Verification items for the finished model (mm, model axes). Face numbers are marked on the shaded views. A direction names the side the tool comes from. Coordinates: 2 decimals unless noted, no trailing zeros. Order: outer loops, then holes, each group sorted by start corner. A loop starts at its lowest first (then second) coordinate and runs counter-clockwise, first axis right, second up. Notation, with made-up numbers: M 79.5,-33.75 L 119.5,-33.75 A11 ccw 119.5,-29.75 Z; hole C 11.25,10 d3. An arc over 180 degrees is marked long. Use one line per item in the form item = value. Start each with the question number.
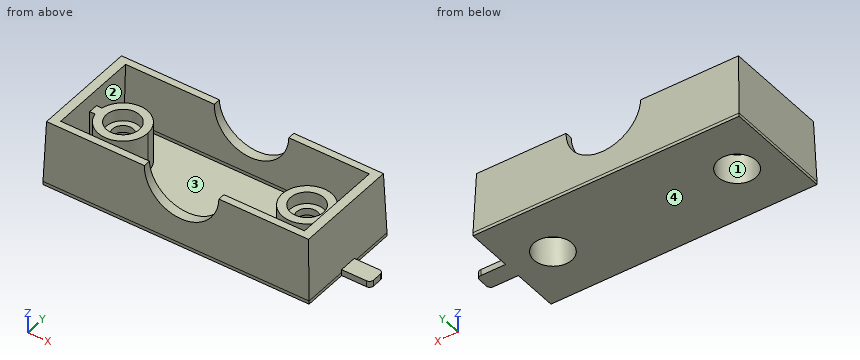
```python
from build123d import *

# Parameters (mm, degrees)
F0_W         = 64.3
F0_H         = 26.3
F1_DEPTH     = 2
F2_W         = 64.3
F2_H         = 26.3
F2_W_2       = 58.9
F2_H_2       = 20.9
F3_DEPTH     = 13.8
F5_DEPTH     = 26.5
F7_DEPTH     = 9.8
F8_R         = 4
F9_DEPTH     = 2.9
F10_R        = 4
F11_DEPTH    = 2.9
F12_R        = 2.5
F13_DEPTH    = 9
F14_R        = 2.5
F15_DEPTH    = 9
F16_R        = 4.6
F17_DEPTH    = 7.2
F18_T1_DEPTH = 102.1483987537
F18_T3_DEPTH = 104.2983987537
F18_T5_DEPTH = 100.1483987537
F19_T1_DEPTH = 53.2490764557
F19_T3_DEPTH = 55.2490764557
F20_W        = 8.1560949282
F20_H        = 4.3
F21_DEPTH    = 1.5
F22_R        = 1


# Not quite as in the source:
# - a fillet or chamfer that OpenCascade refuses, or shapes differently, is made with other operations: its cross-section is extruded or revolved along the edge and cut away or added


with BuildPart() as f1:
    # F0 (on Top) → F1 (new body)
    with BuildSketch(Plane.XY):
        Rectangle(F0_W, F0_H)
    extrude(amount=F1_DEPTH)

    # F2 (on face) → F3 (join)
    with BuildSketch(Plane.XY.offset(2)):
        Rectangle(F2_W, F2_H)
        Rectangle(F2_W_2, F2_H_2, mode=Mode.SUBTRACT)
    extrude(amount=F3_DEPTH)

    # F4 (on face) → F5 (cut)
    with BuildSketch(Plane.XZ.offset(13.15)):
        with BuildLine():
            ThreePointArc((-8, 15.8), (1, 6.8), (10, 15.8))
            Line((10, 15.8), (-8, 15.8))
        make_face()
    extrude(amount=-F5_DEPTH, mode=Mode.SUBTRACT)

    # F6 (on face) → F7 (join)
    with BuildSketch(Plane.XY.offset(2)):
        with BuildLine():
            ThreePointArc((-28.1387604808, -1.15), (-21.6723162131, -5.9721253706), (-16.25, 0))
            ThreePointArc((-16.25, 0), (-21.6723162131, 5.9721253706), (-28.1387604808, 1.15))
            Line((-28.1387604808, 1.15), (-28.1387604808, -1.15))
        make_face()
        with BuildLine():
            Line((-28.1387604808, -1.15), (-28.1387604808, 1.15))
            ThreePointArc((-28.1387604808, 1.15), (-28.25, 0), (-28.1387604808, -1.15))
        make_face()
        with BuildLine():
            ThreePointArc((-28.1387604808, -1.15), (-28.25, 0), (-28.1387604808, 1.15))
            Line((-28.1387604808, 1.15), (-30.8787655085, 1.15))
            Line((-30.8787655085, 1.15), (-30.8787655085, -1.15))
            Line((-30.8787655085, -1.15), (-29.45, -1.15))
            Line((-29.45, -1.15), (-28.1387604808, -1.15))
        make_face()
        with BuildLine():
            ThreePointArc((28.1387604808, -1.15), (28.2221253706, -0.5776837869), (28.25, 0))
            ThreePointArc((28.25, 0), (28.2221253706, 0.5776837869), (28.1387604808, 1.15))
            Line((28.1387604808, 1.15), (28.1387604808, -1.15))
        make_face()
        with BuildLine():
            ThreePointArc((28.1387604808, 1.15), (28.2221253706, 0.5776837869), (28.25, 0))
            ThreePointArc((28.25, 0), (28.2221253706, -0.5776837869), (28.1387604808, -1.15))
            Line((28.1387604808, -1.15), (29.9528725445, -1.15))
            Line((29.9528725445, -1.15), (29.9528725445, 1.15))
            Line((29.9528725445, 1.15), (28.1387604808, 1.15))
        make_face()
        with BuildLine():
            Line((28.1387604808, -1.15), (28.1387604808, 1.15))
            ThreePointArc((28.1387604808, 1.15), (16.25, 0), (28.1387604808, -1.15))
        make_face()
    extrude(amount=F7_DEPTH)

    # F8 (on face) → F9 (cut)
    with BuildSketch(Plane.XY.offset(11.8)):
        with Locations((-22.25, 0)):
            Circle(F8_R)
    extrude(amount=-F9_DEPTH, mode=Mode.SUBTRACT)

    # F10 (on face) → F11 (cut)
    with BuildSketch(Plane.XY.offset(11.8)):
        with Locations((22.25, 0)):
            Circle(F10_R)
    extrude(amount=-F11_DEPTH, mode=Mode.SUBTRACT)

    # F12 (on face) → F13 (cut)
    with BuildSketch(Plane.XY.offset(8.9)):
        with Locations((-22.25, 0)):
            Circle(F12_R)
    extrude(amount=-F13_DEPTH, mode=Mode.SUBTRACT)

    # F14 (on face) → F15 (cut)
    with BuildSketch(Plane.XY.offset(8.9)):
        with Locations((22.25, 0)):
            Circle(F14_R)
    extrude(amount=-F15_DEPTH, mode=Mode.SUBTRACT)

    # F16 (on face) → F17 (cut)
    with BuildSketch(Plane(origin=(0, 0, 0), x_dir=(1, 0, 0), z_dir=(0, 0, -1))):
        with Locations((-22.25, 0)):
            Circle(F16_R)
        with Locations((22.25, 0)):
            Circle(F16_R)
    extrude(amount=-F17_DEPTH, mode=Mode.SUBTRACT)

    # F18: chamfer of 15 x 0.5 on 6 edges, made by hand

    # F18_s2 → F18_t1 (cut)
    with BuildSketch(Plane.YZ.offset(-71.1491993768)):
        Polygon((13.15, 0.8), (12.65, 15.8), (13.15, 15.8), align=None)
        Polygon((-12.65, 15.8), (-13.15, 0.8), (-13.15, 15.8), align=None)
    extrude(amount=F18_T1_DEPTH, mode=Mode.SUBTRACT)

    # F18_s4 → F18_t3 (cut)
    with BuildSketch(Plane.XZ.offset(-52.1491993768)):
        Polygon((32.15, 0.8), (31.65, 15.8), (32.15, 15.8), align=None)
        Polygon((-32.15, 0.8), (-31.65, 15.8), (-32.15, 15.8), align=None)
    extrude(amount=F18_T3_DEPTH, mode=Mode.SUBTRACT)

    # F18_s6 → F18_t5 (cut)
    with BuildSketch(Plane.YZ.offset(-28.9991993768)):
        Polygon((13.15, 0.8), (12.65, 15.8), (13.15, 15.8), align=None)
        Polygon((-12.65, 15.8), (-13.15, 0.8), (-13.15, 15.8), align=None)
    extrude(amount=F18_T5_DEPTH, mode=Mode.SUBTRACT)

    # F19: chamfer of 13 x 0.5 on 4 edges, made by hand

    # F19_s2 → F19_t1 (cut)
    with BuildSketch(Plane.YZ.offset(-23.7990764557)):
        Polygon((-10.95, 15.8), (-10.45, 2.8), (-10.45, 15.8), align=None)
        Polygon((10.45, 2.8), (10.95, 15.8), (10.45, 15.8), align=None)
    extrude(amount=F19_T1_DEPTH, mode=Mode.SUBTRACT)

    # F19_s4 → F19_t3 (cut)
    with BuildSketch(Plane.YZ.offset(-29.45)):
        Polygon((10.45, 2.8), (10.95, 15.8), (10.45, 15.8), align=None)
        Polygon((-10.95, 15.8), (-10.45, 2.8), (-10.45, 15.8), align=None)
    extrude(amount=F19_T3_DEPTH, mode=Mode.SUBTRACT)

    # F20 (on Top) → F21 (join)
    with BuildSketch(Plane.XY):
        with Locations((35.0719525359, 0)):
            Rectangle(F20_W, F20_H)
    extrude(amount=F21_DEPTH)

    # F22
    f22_edges = [f1.edges().sort_by_distance(p)[0] for p in [
        (39.15, 2.15, 0.75),
        (39.15, -2.15, 0.75),
    ]]
    fillet(f22_edges, radius=F22_R)


solid = f1.part
```
1. Tool access check on the marked faces 1 and 2. Record the directions out of +Z, -Z, +X, -X, +Y, -Y that give a thin tool (end or side, any length) a straight path to the whole face; none if there is none.
2. Material ranges on line 1 along X through (y, z) = (2, 4); line 2 along X through (y, z) = (5.5, 5); line 3 along X through (y, z) = (1.5, 11.25), recorded low to high.
3. Cross-section at B-B on x = -22.25. Enter the section's corners in (y, z), and give its area (3 significant figures).
4. Depth check by flat-ended pin: P1, Ø2, axis at x = 15, z = 10, coming from the +Y side; P2, Ø6, axis at y = -1, z = 11, coming from the -X side; P3, Ø4.5, axis at x = 22.5, y = -2, coming from the -Z side; P4, Ø10.5, axis at x = 22.25, y = 0, coming from the -Z side. Enter the tip coordinate at first touch or a pass-through.
5. Cross-section at D-D on x = 24. Enter the section's corners in (y, z).
6. Cross-section at A-A on z = 10.5. Enter the section's corners in (x, y).
7. Cross-section at C-C on x = 1. Enter the section's corners in (y, z).
8. Release check for a two-part mould opening along X. For the marked faces 3 and 4 record: pulls with the +X half, pulls with the -X half, needs draft (parallel to the pull), parting line crosses it, or undercut.
Final values:
q1.face_1 = -Z
q1.face_2 = +Z
q2.line_1 = -32.04 to -29.45, -27.91 to -26.39, -18.11 to -16.59, 16.59 to 18.11, 26.39 to 27.91, 29.45 to 32.04
q2.line_2 = -32.01 to -29.45, -24.65 to -19.85, 19.85 to 24.65, 29.45 to 32.01
q2.line_3 = -31.8 to -29.45, -28.06 to -25.96, -18.54 to -16.44, 16.44 to 18.54, 25.96 to 28.06, 29.45 to 31.8
q3.outline = M -13.15,0 L -4.6,0 L -4.6,7.2 L -2.5,7.2 L -2.5,8.9 L -4,8.9 L -4,11.8 L -6,11.8 L -6,2 L -10.45,2 L -10.45,2.8 L -10.95,15.8 L -12.65,15.8 L -13.15,0.8 Z; M 2.5,7.2 L 4.6,7.2 L 4.6,0 L 13.15,0 L 13.15,0.8 L 12.65,15.8 L 10.95,15.8 L 10.45,2.8 L 10.45,2 L 6,2 L 6,11.8 L 4,11.8 L 4,8.9 L 2.5,8.9 Z
q3.area = 133 mm2
q4.P1 = 12.88
q4.P2 = -31.91
q4.P3 = 7.2
q4.P4 = 0
q5.outline = M -13.15,0 L -4.25,0 L -4.25,7.2 L -1.79,7.2 L -1.79,8.9 L -3.6,8.9 L -3.6,11.8 L -5.74,11.8 L -5.74,2 L -10.45,2 L -10.45,2.8 L -10.95,15.8 L -12.65,15.8 L -13.15,0.8 Z; M 1.79,7.2 L 4.25,7.2 L 4.25,0 L 13.15,0 L 13.15,0.8 L 12.65,15.8 L 10.95,15.8 L 10.45,2.8 L 10.45,2 L 5.74,2 L 5.74,11.8 L 3.6,11.8 L 3.6,8.9 L 1.79,8.9 Z
q6.outline = M -31.83,-12.83 L -6.27,-12.83 L -6.27,-10.75 L -29.45,-10.75 L -29.45,-1.15 L -28.14,-1.15 A6 ccw long -28.14,1.15 L -29.45,1.15 L -29.45,10.75 L -6.27,10.75 L -6.27,12.83 L -31.83,12.83 Z; M 8.27,-12.83 L 31.83,-12.83 L 31.83,12.83 L 8.27,12.83 L 8.27,10.75 L 29.45,10.75 L 29.45,1.15 L 28.14,1.15 A6 ccw long 28.14,-1.15 L 29.45,-1.15 L 29.45,-10.75 L 8.27,-10.75 Z; hole C -22.25,0 d8; hole C 22.25,0 d8
q7.outline = M -13.15,0 L 13.15,0 L 13.15,0.8 L 12.95,6.8 L 10.6,6.8 L 10.45,2.8 L 10.45,2 L -10.45,2 L -10.45,2.8 L -10.6,6.8 L -12.95,6.8 L -13.15,0.8 Z
q8.face_3 = undercut
q8.face_4 = needs draft
